from build123d import *

# Parameters (mm, degrees)
ESQUISSE1_R             = 1.5
BOSS_EXTRU_1_DEPTH      = 16.5
ESQUISSE2_R             = 2
BOSS_EXTRU_2_DEPTH      = 2
ESQUISSE3_W             = 1
ESQUISSE3_H             = 4
ENL_V_MAT_EXTRU_1_DEPTH = 1
CONG_1_R                = 0.5


with BuildPart() as part:
    # Esquisse1 → Boss.-Extru.1 (new body)
    with BuildSketch(Plane(origin=(0, 0, 0), x_dir=(1, 0, 0), z_dir=(0, 1, 0))):
        Circle(ESQUISSE1_R)
    extrude(amount=BOSS_EXTRU_1_DEPTH)

    # Esquisse2 → Boss.-Extru.2 (add)
    with BuildSketch(Plane(origin=(0, 16.5, 0), x_dir=(1, 0, 0), z_dir=(0, 1, 0))):
        Circle(ESQUISSE2_R)
    extrude(amount=BOSS_EXTRU_2_DEPTH)

    # Esquisse3 → Enlèv. mat.-Extru.1 (cut)
    with BuildSketch(Plane(origin=(0, 18.5, 0), x_dir=(1, 0, 0), z_dir=(0, 1, 0))):
        Rectangle(ESQUISSE3_W, ESQUISSE3_H)
    extrude(amount=-ENL_V_MAT_EXTRU_1_DEPTH, mode=Mode.SUBTRACT)

    # Congé1
    cong_1_edges = [part.edges().sort_by_distance(p)[0] for p in [
        (1.58113883, 18.5, -1.224744871),
        (-2, 18.5, 0),
    ]]
    fillet(cong_1_edges, radius=CONG_1_R)


solid = part.part
Can you work these out from the model? Positions are in its coordinate system, mm. A direction names the side the tool comes from. Round coordinates to 2 decimals unless told otherwise and drop trailing zeros. Loops run counter-clockwise (first coordinate to the right, second up) from the corner with the lowest first, then second, coordinate; pieces in that order, holes last. Notation, with made-up numbers: (-10, 34.25) - (-2, 34.25) arc R36 cw to (-2, 71.25) - close; hole circle Ø5 at (59, 29). An arc over 180 degrees is marked (long way). Answer in a Markdown table with one row per item. Add a question column.
Q1. For pin 1 Ø0.8 at (y, z) = (18, -0.5) entering from -X; pin 2 Ø0.8 at (y, z) = (18, 0.5) entering from +X, each with a flat end and sliding along its axis, tell me the tip position at first contact or that it passes through.
Q2. I want a section at B-B on x = 0. List the corners of the cut face in (y, z) for me.
Q3. Which directions (+Z, -Z, +X, -X, +Y, -Y) give clear straight access to the entire face, cutting with the end or side of a thin tool? Please do faces 1 (the cylindrical face through (1.847, 17.24, 0.766)), 2 (the flat face through (0.5, 18, 0)), 3 (the cylindrical face through (-1.5, 8.13, -0.07)).
Q4. I need wall thicknesses on L1, parallel to Y at x = -0.1, z = 0.3; L2, parallel to X at y = 15.25, z = 0; L3, parallel to Z at x = -1.25, y = 12.5. Which ranges of each line are inside material? Lowest first, please.
Q5. I want a section at A-A on z = 0. List the corners of the cut face in (x, y) for me.
Q6. I want a section at C-C on y = 7. List the corners of the cut face in (x, z) for me.
A:
| question | item | result |
|---|---|---|
| 1 | pin 1 | x = -2 |
| 1 | pin 2 | x = 2 |
| 2 | outline | (0, -1.5) - (16.5, -1.5) - (16.5, -2) - (17.5, -2) - (17.5, 2) - (16.5, 2) - (16.5, 1.5) - (0, 1.5) - close |
| 3 | face 1 | +Y, -Y |
| 3 | face 2 | +Z, -Z, +Y |
| 3 | face 3 | -Y |
| 4 | L1 | 0 to 17.5 |
| 4 | L2 | -1.5 to 1.5 |
| 4 | L3 | -0.83 to 0.83 |
| 5 | outline | (-2, 16.5) - (-1.5, 16.5) - (-1.5, 0) - (1.5, 0) - (1.5, 16.5) - (2, 16.5) - (2, 18) arc R0.5 ccw to (1.5, 18.5) - (0.5, 18.5) - (0.5, 17.5) - (-0.5, 17.5) - (-0.5, 18.5) - (-1.5, 18.5) arc R0.5 ccw to (-2, 18) - close |
| 6 | outline | circle Ø3 at (0, 0) |
